```python
from build123d import *

# Parameters (mm, degrees)
F1_DEPTH = 177.8
F2_R     = 5


with BuildPart() as f1:
    # F0 (on Front) → F1 (new body)
    with BuildSketch(Plane.XZ):
        with BuildLine():
            Line((195, 0), (5, 0))
            ThreePointArc((5, 0), (1.4644660941, -1.4644660941), (0, -5))
            Line((0, -5), (0, -97))
            Line((0, -97), (-25.9807621135, -142))
            Line((-25.9807621135, -142), (-23.6857947935, -143.325))
            Line((-23.6857947935, -143.325), (2.65, -97.7100653599))
            Line((2.65, -97.7100653599), (2.65, -5))
            ThreePointArc((2.65, -5), (3.3382990642, -3.3382990642), (5, -2.65))
            Line((5, -2.65), (195, -2.65))
            ThreePointArc((195, -2.65), (196.6617009358, -3.3382990642), (197.35, -5))
            Line((197.35, -5), (197.35, -97.7100653599))
            Line((197.35, -97.7100653599), (223.6857947935, -143.325))
            Line((223.6857947935, -143.325), (225.9807621135, -142))
            Line((225.9807621135, -142), (200, -97))
            Line((200, -97), (200, -5))
            ThreePointArc((200, -5), (198.5355339059, -1.4644660941), (195, 0))
        make_face()
    extrude(amount=F1_DEPTH)

    # F2
    f2_edges = [f1.edges().sort_by_distance(p)[0] for p in [
        (200, -88.9, -97),
        (197.35, -88.9, -97.710065),
        (2.65, -88.9, -97.710065),
        (0, -88.9, -97),
    ]]
    fillet(f2_edges, radius=F2_R)


solid = f1.part
```
Design review of the part built by this model. Coordinates are the model's own, in mm. A direction names the side the tool comes from. Give positions to 0.01 mm unless a question says otherwise; leave off trailing zeros. Write each loop counter-clockwise with the first axis right and the second up, starting at its lowest first coordinate (ties: lowest second). Pieces come first, ordered by that corner, then holes. Notation, with made-up numbers: (-38.75, -37) -> (-28.75, -37) arc R23 cw to (-28.75, -27) -> close; hole circle Ø4 at (5.25, 20.25). An arc over 180 degrees is marked (long way). Answer in a Markdown table with one row per item.
(1) Mouldability with a two-part tool opening along X and no side actions: class faces 4 (the flat face through (2.65, -88, -51)), 5 (the flat face through (-13.148, -87.655, -119.773)), 6 (the flat face through (99, 0, -2)) as +X half, -X half, draft (parallel to the pull), parting line (faces both ways), or undercut.
Results:
| item | result |
|---|---|
| face 4 | undercut |
| face 5 | -X half |
| face 6 | draft |
(2) Consider section A-A (z = -25). State the section outline as (x, y) points, then the cut area to 3 significant figures.
Results:
| item | result |
|---|---|
| outline | (0, -177.8) -> (2.65, -177.8) -> (2.65, 0) -> (0, 0) -> close; (197.35, -177.8) -> (200, -177.8) -> (200, 0) -> (197.35, 0) -> close |
| area | 942 mm2 |
(3) Consider section C-C (x = 168). State the section outline as (y, z) points.
Results:
| item | result |
|---|---|
| outline | (-177.8, -2.65) -> (0, -2.65) -> (0, 0) -> (-177.8, 0) -> close |
(4) For faces 1 (the flat face through (0, -88, -50)), 2 (the flat face through (200, -88, -51)), 3 (the flat face through (-11.032, -87.655, -121.409)), list the 3-axis set-ups (+Z, -Z, +X, -X, +Y, -Y) from which the entire face can be reached by the end or side of a thin tool; tool diameter is ignored.
Results:
| item | result |
|---|---|
| face 1 | +Z, -X, +Y, -Y |
| face 2 | +Z, +X, +Y, -Y |
| face 3 | -Z, +Y, -Y |
(5) Consider section D-D (z = -127.5). State the section outline as (x, y) points.
Results:
| item | result |
|---|---|
| outline | (-17.61, -177.8) -> (-14.55, -177.8) -> (-14.55, 0) -> (-17.61, 0) -> close; (214.55, -177.8) -> (217.61, -177.8) -> (217.61, 0) -> (214.55, 0) -> close |
(6) Consider section B-B (y = -77.5). State the section outline as (x, z) points (3 decimals), then the cut area to 3 significant figures.
Results:
| item | result |
|---|---|
| outline | (-25.981, -142) -> (-23.686, -143.325) -> (1.98, -98.87) arc R5 ccw to (2.65, -96.37) -> (2.65, -5) arc R2.35 cw to (5, -2.65) -> (195, -2.65) arc R2.35 cw to (197.35, -5) -> (197.35, -96.37) arc R5 ccw to (198.02, -98.87) -> (223.686, -143.325) -> (225.981, -142) -> (200.67, -98.16) arc R5 cw to (200, -95.66) -> (200, -5) arc R5 ccw to (195, 0) -> (5, 0) arc R5 ccw to (0, -5) -> (0, -95.66) arc R5 cw to (-0.67, -98.16) -> close |
| area | 1,300 mm2 |
(7) Clearance check with flat-ended pins moving along their axes: pin 1 (8 mm diameter, centred on y = -42.5, z = -111.5, fed in from +X); pin 2 (2 mm diameter, centred on y = -150.5, z = -88, fed in from -X); pin 3 (2 mm diameter, centred on x = 91, y = -89.5, fed in from -Z). State where each tip first meets the part, or that it passes through.
Results:
| item | result |
|---|---|
| pin 1 | x = 210.68 |
| pin 2 | x = 0 |
| pin 3 | z = -2.65 |
(8) To check wall thickness, follow probe 1 along X at (y, z) = (-80, -43.5); probe 2 along Z at (x, y) = (128, -41). State the ranges of each line that lie inside material, in increasing order.
Results:
| item | result |
|---|---|
| probe 1 | 0 to 2.65, 197.35 to 200 |
| probe 2 | -2.65 to 0 |
